from build123d import *

# Parameters (mm, degrees)
BOSS_EXTRU_1_DEPTH      = 19
ESQUISSE2_R             = 1.7
BOSS_EXTRU_8_DEPTH      = 4.5
ESQUISSE2_4_R           = 1.7
BOSS_EXTRU_9_DEPTH      = 3
ESQUISSE5_W             = 15
ESQUISSE5_H             = 4.5
ENL_V_MAT_EXTRU_1_DEPTH = 1.75
ESQUISSE20_W            = 19
ESQUISSE20_H            = 3.718185323
BOSS_EXTRU_18_DEPTH     = 3
ESQUISSE21_W            = 3
ESQUISSE21_H            = 19
BOSS_EXTRU_19_DEPTH     = 40
ESQUISSE22_W            = 19
ESQUISSE22_H            = 4
BOSS_EXTRU_20_DEPTH     = 3
ESQUISSE23_W            = 6
ESQUISSE23_H            = 4
BOSS_EXTRU_21_DEPTH     = 19.3
ESQUISSE24_W            = 1.75
ESQUISSE24_H            = 4
BOSS_EXTRU_22_DEPTH     = 33
ESQUISSE25_W            = 2
ESQUISSE25_H            = 4.324516653
ENL_V_MAT_EXTRU_6_DEPTH = 1.75
ESQUISSE26_W            = 3.2
ESQUISSE26_H            = 1.5
BOSS_EXTRU_23_DEPTH     = 5
ESQUISSE27_W            = 1.5
ESQUISSE27_H            = 5
BOSS_EXTRU_24_DEPTH     = 3.7
BOSS_EXTRU_26_REACH     = 63.655
ESQUISSE29_W            = 3
ESQUISSE29_H            = 19
ESQUISSE30_W            = 1.499569939
ESQUISSE30_H            = 10
BOSS_EXTRU_27_DEPTH     = 36
ESQUISSE31_W            = 3
ESQUISSE31_H            = 36.935070483
ENL_V_MAT_EXTRU_7_DEPTH = 9
ESQUISSE32_W            = 3
ESQUISSE32_H            = 9
BOSS_EXTRU_28_DEPTH     = 7.5
ESQUISSE33_W            = 6.9
ESQUISSE33_H            = 1.5
BOSS_EXTRU_29_DEPTH     = 28
ESQUISSE34_W            = 6.9
ESQUISSE34_H            = 4.363408043
BOSS_EXTRU_30_DEPTH     = 22.475483347
ESQUISSE35_W            = 2.65
ESQUISSE35_H            = 4.363408043
BOSS_EXTRU_31_DEPTH     = 10
ESQUISSE36_W            = 2
ESQUISSE36_H            = 4
BOSS_EXTRU_32_DEPTH     = 6.5
ESQUISSE37_W            = 1.75
ESQUISSE37_H            = 34.75
BOSS_EXTRU_33_DEPTH     = 2


with BuildPart() as part:
    # Esquisse1 → Boss.-Extru.1 (new body)
    with BuildSketch(Plane.XY):
        with BuildLine():
            Line((-10.5, -11.806354221), (-10.5, -19.242724867))
            Line((-10.5, -19.242724867), (10.5, -19.242724867))
            Line((10.5, -19.242724867), (10.5, -11.806354221))
            ThreePointArc((10.5, -11.806354221), (0, 15.8), (-10.5, -11.806354221))
        make_face()
        with BuildLine():
            Line((-8.75, -10.992724867), (-8.75, -17.492724867))
            Line((-8.75, -17.492724867), (8.75, -17.492724867))
            Line((8.75, -17.492724867), (8.75, -10.992724867))
            ThreePointArc((8.75, -10.992724867), (0, 14.05), (-8.75, -10.992724867))
        make_face(mode=Mode.SUBTRACT)
    extrude(amount=BOSS_EXTRU_1_DEPTH)



with BuildPart() as body_2:
    # Esquisse2 → Boss.-Extru.8 (new body)
    # profile 1 of 4: a face of its own
    with BuildSketch(Plane.XY.offset(19)):
        with BuildLine():
            ThreePointArc((-15.8, 0), (-15.70155977, 1.760971547), (-15.407465723, 3.5))
            Line((-15.407465723, 3.5), (-17.095274292, 3.5))
            ThreePointArc((-17.095274292, 3.5), (-19.561128115, 2.473312424), (-20.569715298, 0))
            ThreePointArc((-20.569715298, 0), (-19.561128115, -2.473312424), (-17.095274292, -3.5))
            Line((-17.095274292, -3.5), (-15.407465723, -3.5))
            ThreePointArc((-15.407465723, -3.5), (-15.70155977, -1.760971547), (-15.8, 0))
        make_face()
        with Locations((-17.5, 0)):
            Circle(ESQUISSE2_R, mode=Mode.SUBTRACT)
    # profile 2 of 4: a face of its own
    with BuildSketch(Plane.XY.offset(19)):
        with BuildLine():
            Line((17.095274292, 3.5), (15.407465723, 3.5))
            ThreePointArc((15.407465723, 3.5), (15.70155977, 1.76097155), (15.8, 5e-09))
            ThreePointArc((15.8, 5e-09), (15.70155977, -1.760971545), (15.407465723, -3.5))
            Line((15.407465723, -3.5), (17.095274292, -3.5))
            ThreePointArc((17.095274292, -3.5), (19.561128115, -2.473312424), (20.569715298, 0))
            ThreePointArc((20.569715298, 0), (19.561128115, 2.473312424), (17.095274292, 3.5))
        make_face()
        with BuildLine():
            ThreePointArc((19.2, 0), (17.499999997, -1.7), (15.8, 5e-09))
            ThreePointArc((15.8, 5e-09), (17.500000003, 1.7), (19.2, 0))
        make_face(mode=Mode.SUBTRACT)
    # profile 3 of 4: a face of its own
    with BuildSketch(Plane.XY.offset(19)):
        with Locations((-17.5, 0)):
            Circle(ESQUISSE2_R)
    # profile 4 of 4: a face of its own
    with BuildSketch(Plane.XY.offset(19)):
        with Locations((17.5, 0)):
            Circle(ESQUISSE2_R)
    extrude(amount=-BOSS_EXTRU_8_DEPTH)


with BuildPart() as part_1:
    add(part.part)

    add(body_2.part)  # Boss.-Extru.9 merges body 2
    # Esquisse2<4> → Boss.-Extru.9 (add)
    with BuildSketch(Plane.XY.offset(19)):
        with Locations((-17.5, 0)):
            Circle(ESQUISSE2_4_R)
        with Locations((17.5, 0)):
            Circle(ESQUISSE2_4_R)
    extrude(amount=BOSS_EXTRU_9_DEPTH)

    # Esquisse5 → Enlèv. mat.-Extru.1 (cut)
    with BuildSketch(Plane.XZ.offset(19.242724867)):
        with Locations((0, 16.75)):
            Rectangle(ESQUISSE5_W, ESQUISSE5_H)
    extrude(amount=-ENL_V_MAT_EXTRU_1_DEPTH, mode=Mode.SUBTRACT)

    # Esquisse20 → Boss.-Extru.18 (add)
    with BuildSketch(Plane.ZY.offset(10.5)):
        with Locations((9.5, -17.383632205)):
            Rectangle(ESQUISSE20_W, ESQUISSE20_H)
    extrude(amount=BOSS_EXTRU_18_DEPTH)

    # Esquisse21 → Boss.-Extru.19 (add)
    with BuildSketch(Plane.XZ.offset(19.242724867)):
        with Locations((-12, 9.5)):
            Rectangle(ESQUISSE21_W, ESQUISSE21_H)
    extrude(amount=BOSS_EXTRU_19_DEPTH)

    # Esquisse22 → Boss.-Extru.20 (add)
    with BuildSketch(Plane(origin=(-10.5, 0, 0), x_dir=(0, 0, -1), z_dir=(1, 0, 0))):
        with Locations((-9.5, -57.242724867)):
            Rectangle(ESQUISSE22_W, ESQUISSE22_H)
    extrude(amount=BOSS_EXTRU_20_DEPTH)

    # Esquisse23 → Boss.-Extru.21 (add)
    with BuildSketch(Plane.XY.offset(19)):
        with Locations((-10.5, -57.242724867)):
            Rectangle(ESQUISSE23_W, ESQUISSE23_H)
    extrude(amount=BOSS_EXTRU_21_DEPTH)

    # Esquisse24 → Boss.-Extru.22 (add)
    with BuildSketch(Plane(origin=(0, -55.242724867, 0), x_dir=(1, 0, 0), z_dir=(0, 1, 0))):
        with Locations((-8.375, -36.3)):
            Rectangle(ESQUISSE24_W, ESQUISSE24_H)
    extrude(amount=BOSS_EXTRU_22_DEPTH)

    # Esquisse25 → Enlèv. mat.-Extru.6 (cut)
    with BuildSketch(Plane(origin=(0, -55.242724867, 0), x_dir=(1, 0, 0), z_dir=(0, 1, 0))):
        with Locations((-10.25, -36.137741674)):
            Rectangle(ESQUISSE25_W, ESQUISSE25_H)
    extrude(amount=-ENL_V_MAT_EXTRU_6_DEPTH, mode=Mode.SUBTRACT)

    # Esquisse26 → Boss.-Extru.23 (add)
    with BuildSketch(Plane(origin=(0, -55.242724867, 0), x_dir=(1, 0, 0), z_dir=(0, 1, 0))):
        with Locations((-10.85, -33.225483347)):
            Rectangle(ESQUISSE26_W, ESQUISSE26_H)
    extrude(amount=BOSS_EXTRU_23_DEPTH)

    # Esquisse27 → Boss.-Extru.24 (add)
    with BuildSketch(Plane.ZY.offset(12.45)):
        with Locations((33.225483347, -52.742724867)):
            Rectangle(ESQUISSE27_W, ESQUISSE27_H)
    extrude(amount=BOSS_EXTRU_24_DEPTH)

    # Esquisse29 → Boss.-Extru.26 (add, up to next)
    with BuildSketch(Plane(origin=(0, -15.524539544, 0), x_dir=(1, 0, 0), z_dir=(0, 1, 0)), mode=Mode.PRIVATE) as boss_extru_26_sk1:
        with Locations((-12, -9.5)):
            Rectangle(ESQUISSE29_W, ESQUISSE29_H)
    boss_extru_26_tool1 = extrude(boss_extru_26_sk1.sketch, amount=BOSS_EXTRU_26_REACH, mode=Mode.PRIVATE) - part_1.part
    add(boss_extru_26_tool1.solids().sort_by_distance((-12, -15.52454, 9.5))[0])

    # Esquisse30 → Boss.-Extru.27 (add)
    with BuildSketch(Plane.XZ.offset(19.242724867)):
        with Locations((-9.750215031, 5)):
            Rectangle(ESQUISSE30_W, ESQUISSE30_H)
    extrude(amount=BOSS_EXTRU_27_DEPTH)

    # Esquisse31 → Enlèv. mat.-Extru.7 (cut)
    with BuildSketch(Plane.XY.offset(19)):
        with Locations((-12, -40.258799307)):
            Rectangle(ESQUISSE31_W, ESQUISSE31_H)
    extrude(amount=-ENL_V_MAT_EXTRU_7_DEPTH, mode=Mode.SUBTRACT)

    # Esquisse32 → Boss.-Extru.28 (add)
    with BuildSketch(Plane(origin=(0, -58.726334549, 0), x_dir=(1, 0, 0), z_dir=(0, 1, 0))):
        with Locations((-12, -14.5)):
            Rectangle(ESQUISSE32_W, ESQUISSE32_H)
    extrude(amount=BOSS_EXTRU_28_DEPTH)

    # Esquisse33 → Boss.-Extru.29 (add)
    with BuildSketch(Plane(origin=(0, -50.242724867, 0), x_dir=(1, 0, 0), z_dir=(0, 1, 0))):
        with Locations((-12.7, -33.225483347)):
            Rectangle(ESQUISSE33_W, ESQUISSE33_H)
    extrude(amount=BOSS_EXTRU_29_DEPTH)

    # Esquisse34 → Boss.-Extru.30 (add)
    with BuildSketch(Plane(origin=(0, 0, 32.475483347), x_dir=(-1, 0, 0), z_dir=(0, 0, -1))):
        with Locations((12.7, -34.093482268)):
            Rectangle(ESQUISSE34_W, ESQUISSE34_H)
    extrude(amount=BOSS_EXTRU_30_DEPTH)

    # Esquisse35 → Boss.-Extru.31 (add)
    with BuildSketch(Plane(origin=(0, 0, 10), x_dir=(-1, 0, 0), z_dir=(0, 0, -1))):
        with Locations((14.825, -34.093482268)):
            Rectangle(ESQUISSE35_W, ESQUISSE35_H)
    extrude(amount=BOSS_EXTRU_31_DEPTH)

    # Esquisse36 → Boss.-Extru.32 (add)
    with BuildSketch(Plane.XY.offset(33.975483347)):
        with Locations((-15.15, -26.925726739)):
            Rectangle(ESQUISSE36_W, ESQUISSE36_H)
        with Locations((-15.15, -34.925726739)):
            Rectangle(ESQUISSE36_W, ESQUISSE36_H)
        with Locations((-15.15, -42.925726739)):
            Rectangle(ESQUISSE36_W, ESQUISSE36_H)
        with Locations((-15.15, -50.925726739)):
            Rectangle(ESQUISSE36_W, ESQUISSE36_H)
    extrude(amount=BOSS_EXTRU_32_DEPTH)

    # Esquisse37 → Boss.-Extru.33 (add)
    with BuildSketch(Plane.XY.offset(38.3)):
        with Locations((-8.375, -39.617724867)):
            Rectangle(ESQUISSE37_W, ESQUISSE37_H)
    extrude(amount=BOSS_EXTRU_33_DEPTH)


solid = part_1.part
Here's how the part is built. I have some questions about the finished solid (model axes, mm). A direction names the side the tool comes from. Round coordinates to 2 decimals unless told otherwise and drop trailing zeros. Loops run counter-clockwise (first coordinate to the right, second up) from the corner with the lowest first, then second, coordinate; pieces in that order, holes last. Notation, with made-up numbers: (-37.75, 54) -> (14.25, 54) arc R11 ccw to (14.25, 69) -> close; hole circle Ø4 at (29, 70). An arc over 180 degrees is marked (long way). Write each question's results on one line, items separated by ' | '.
(1) If we section it at B-B, the plane z = 29.5: List the corners of the cut face in (x, y) for me.
Worked answers:
outline: (-16.15, -36.28) -> (-9.25, -36.28) -> (-9.25, -31.91) -> (-16.15, -31.91) -> close; (-13.5, -59.24) -> (-7.5, -59.24) -> (-7.5, -55.24) -> (-13.5, -55.24) -> close
(2) We'd pull the mould along Y, two halves only. Please class faces 1 (the face through (-12, -53, 19)), 2 (the face through (-11, -59.243, 19)), 3 (the face through (18, 0, 14.5)): released by +Y, released by -Y, zero draft, split by the parting line, or undercut.
Worked answers:
face 1: undercut | face 2: released by -Y | face 3: zero draft
(3) For faces 4 (the face through (-13, -46, 32.475)), 5 (the face through (10.5, -16, 9)), 6 (the face through (-9.25, -35, 26)), 7 (the face through (-14.15, -35, 37)), 8 (the face through (-12, -21.791, 15)), which set-ups out of +Z, -Z, +X, -X, +Y, -Y let a thin tool reach every point of the face, with its end or its side?
Worked answers:
face 4: +X, -X | face 5: +Z, -Z, +X, -Y | face 6: +X | face 7: +Z, +Y, -Y | face 8: +Z, +X, -X
(4) If we section it at A-A, the plane y = -34.5: List the corners of the cut face in (x, z) for me, then the cut area to 3 significant figures.
Worked answers:
outline: (-16.15, 0) -> (-9, 0) -> (-9, 10) -> (-9.25, 10) -> (-9.25, 33.98) -> (-14.15, 33.98) -> (-14.15, 40.48) -> (-16.15, 40.48) -> close; (-9.25, 34.3) -> (-7.5, 34.3) -> (-7.5, 40.3) -> (-9.25, 40.3) -> close | area: 260 mm2
(5) For P1, Ø1.9, axis at x = -16.5, z = 17.5, coming from the +Y side; P2, Ø6.5, axis at x = -12, z = 8.5, coming from the +Y side; P3, Ø15, axis at y = -23, z = 13, coming from the -X side; P4, Ø7, axis at y = -44.5, z = 27, coming from the +X side, each with a flat end and sliding along its axis, tell me the tip position at first contact or that it passes through.
Worked answers:
P1: y = 3.5 | P2: y = 13.16 | P3: x = -13.5 | P4: through
(6) If we section it at D-D, the plane z = 20: List the corners of the cut face in (x, y) for me.
Worked answers:
outline: circle Ø3.4 at (-17.5, 0); (-16.15, -36.28) -> (-9.25, -36.28) -> (-9.25, -31.91) -> (-16.15, -31.91) -> close; (-13.5, -59.24) -> (-7.5, -59.24) -> (-7.5, -55.24) -> (-13.5, -55.24) -> close; circle Ø3.4 at (17.5, 0)
(7) If we section it at C-C, the plane x = -4: List the corners of the cut face in (y, z) for me, then the cut area to 3 significant figures.
Worked answers:
outline: (-19.24, 0) -> (-17.49, 0) -> (-17.49, 14.5) -> (-19.24, 14.5) -> close; (13.47, 0) -> (15.29, 0) -> (15.29, 19) -> (13.47, 19) -> close | area: 59.9 mm2
(8) If I drill on L1, parallel to X at y = 0, z = 8.75; L2, parallel to Y at x = 0, z = 4; L3, parallel to Y at x = -10, z = 17.5, over which ranges is the centre line in solid material (lowest first)?
Worked answers:
L1: -15.8 to -14.05, 14.05 to 15.8 | L2: -19.24 to -17.49, 14.05 to 15.8 | L3: -59.24 to -55.24, -36.28 to -31.91, -19.24 to -9.87, 9.87 to 12.23
